Check sheet for the modelled part. Datum: model origin and axes. Units: mm. Face numbers are marked on the shaded views. Round coordinates to 2 decimals unless told otherwise and drop trailing zeros. Write each loop counter-clockwise with the first axis right and the second up, starting at its lowest first coordinate (ties: lowest second). Pieces come first, ordered by that corner, then holes. Notation, with made-up numbers: (1.5, 15.25) -> (33.5, 15.25) arc R7 ccw to (33.5, 25.25) -> close; hole circle Ø11 at (70, 53.25). An arc over 180 degrees is marked (long way). One line per item, written item: value.
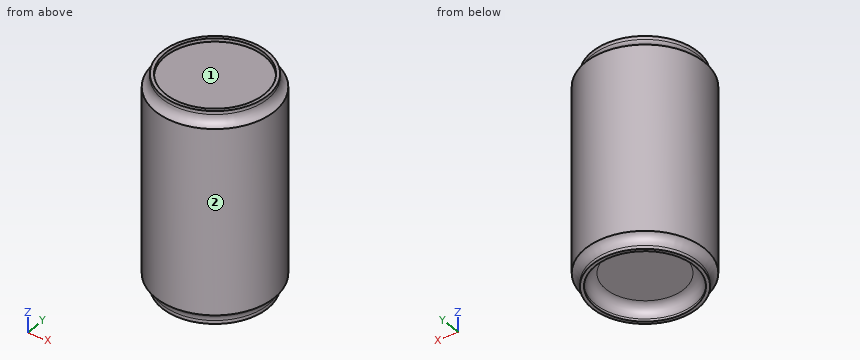
from build123d import *

# Parameters (mm, degrees)
F0_R     = 28.575
F0_R_2   = 25.4
F1_DEPTH = 95.25
F0_R_3   = 23.8125
F2_DEPTH = 101.6
F3_DEPTH = 6.35
F4_DEPTH = 100.0125
F5_DEPTH = 6.35
F6_DEPTH = 6.35
F7_R     = 5.08
F9_T     = -2.54


# Not quite as in the source:
# - a fillet or chamfer that OpenCascade refuses, or shapes differently, is made with other operations: its cross-section is extruded or revolved along the edge and cut away or added


with BuildPart() as f1:
    # F0 (on Top) → F1 (new body)
    with BuildSketch(Plane.XY):
        Circle(F0_R)
        Circle(F0_R_2, mode=Mode.SUBTRACT)
    extrude(amount=F1_DEPTH)

    # F0 (on Top) → F2 (join)
    with BuildSketch(Plane.XY):
        Circle(F0_R_2)
        Circle(F0_R_3, mode=Mode.SUBTRACT)
    extrude(amount=F2_DEPTH)

    # F0 (on Top) → F3 (cut)
    with BuildSketch(Plane.XY):
        Circle(F0_R)
        Circle(F0_R_2, mode=Mode.SUBTRACT)
    extrude(amount=F3_DEPTH, mode=Mode.SUBTRACT)

    # F0 (on Top) → F4 (join)
    with BuildSketch(Plane.XY):
        Circle(F0_R_3)
    extrude(amount=F4_DEPTH)

    # F0 (on Top) → F5 (join)
    with BuildSketch(Plane.XY):
        Circle(F0_R_3)
    extrude(amount=F5_DEPTH)

    # F0 (on Top) → F6 (cut)
    with BuildSketch(Plane.XY):
        Circle(F0_R_3)
    extrude(amount=F6_DEPTH, mode=Mode.SUBTRACT)

    # F7
    f7_edges = [f1.edges().sort_by_distance(p)[0] for p in [
        (-23.8125, 0, 6.35),
    ]]
    fillet(f7_edges, radius=F7_R)

    # F8: fillet of radius 5.08 on 2 edges, made by hand

    # F8_s1 → F8_t2 (revolve)
    with BuildSketch(Plane.XZ):
        with BuildLine():
            ThreePointArc((25.4, 1.6407139607), (26.2678865162, 4.4805202921), (28.575, 6.35))
            Line((28.575, 6.35), (25.4, 6.35))
            Line((25.4, 6.35), (25.4, 1.6407139607))
        make_face()
    revolve(axis=Axis((0, 0, 6.35), (0, 0, 1)))

    # F8_s3 → F8_t4 (revolve)
    with BuildSketch(Plane.XZ):
        with BuildLine():
            ThreePointArc((28.575, 95.25), (26.2678865162, 97.1194797079), (25.4, 99.9592860393))
            Line((25.4, 99.9592860393), (25.4, 95.25))
            Line((25.4, 95.25), (28.575, 95.25))
        make_face()
    revolve(axis=Axis((0, 0, 95.25), (0, 0, 1)))

    # F9 (hollow: no face is removed)
    offset(amount=F9_T, mode=Mode.SUBTRACT)


solid = f1.part
Item 1: Sectioned sample at C-C (z = 85). Enter the section's corners in (x, y) (3 decimals).
Result set:
outline: circle Ø57.15 at (0, 0); hole circle Ø52.07 at (0, 0)
Item 2: Depth check by flat-ended pin: pin 1 (4 mm diameter, centred on x = 1.5, z = 29, fed in from +Y) (3 decimals); pin 2 (8 mm diameter, centred on x = -16.5, y = 1, fed in from -Z); pin 3 (4 mm diameter, centred on x = -19.5, z = 54.5, fed in from +Y); pin 4 (10 mm diameter, centred on y = -2.5, z = 29.5, fed in from +X) (3 decimals). Enter the tip coordinate at first touch or a pass-through.
Result set:
pin 1: y = 28.575
pin 2: z = 6.02
pin 3: y = 22.59
pin 4: x = 28.575
Item 3: Release check for a two-part mould opening along X. For the marked faces 1 and 2 record: pulls with the +X half, pulls with the -X half, needs draft (parallel to the pull), parting line crosses it, or undercut.
Result set:
face 1: undercut
face 2: parting line crosses it
Item 4: Material ranges on line 1 along Y through (x, z) = (0, 0.8); line 2 along X through (y, z) = (0.5, 28.5); line 3 along Y through (x, z) = (0, 72.5) (3 decimals), recorded low to high.
Result set:
line 1: -25.4 to -23.81, 23.81 to 25.4
line 2: -28.57 to -26.03, 26.03 to 28.57
line 3: -28.575 to -26.035, 26.035 to 28.575
